Design review of the part built by this model. Coordinates are the model's own, in mm. A direction names the side the tool comes from. Coordinates: 2 decimals unless noted, no trailing zeros. Write each loop counter-clockwise with the first axis right and the second up, starting at its lowest first coordinate (ties: lowest second). Pieces come first, ordered by that corner, then holes. Notation, with made-up numbers: (-20.75, 2) - (-0.75, 2) arc R12 ccw to (-0.75, 11) - close; hole circle Ø1 at (71, 45). An arc over 180 degrees is marked (long way). One line per item, written item: value.
from build123d import *

# Parameters (mm, degrees)
ESBO_O1_W                  = 27
ESBO_O1_H                  = 75
RESSALTO_EXTRUS_O1_DEPTH   = 2
ESBO_O2_W                  = 75
ESBO_O2_H                  = 104
RESSALTO_EXTRUS_O2_DEPTH   = 2
ESBO_O3_W                  = 29
ESBO_O3_H                  = 75
RESSALTO_EXTRUS_O3_DEPTH   = 2
ESBO_O4_R                  = 5
CORTE_EXTRUS_O1_DEPTH      = 2
ESBO_O5_R                  = 2.5
CORTE_EXTRUS_O2_DEPTH      = 1
CORTE_EXTRUS_O2_DEPTH_BACK = 107
ESBO_O7_R                  = 3.5
CORTE_EXTRUS_O3_DEPTH      = 10


with BuildPart() as part:
    # Esboço1 → Ressalto-extrusão1 (new body)
    with BuildSketch(Plane(origin=(0, 0, 0), x_dir=(1, 0, 0), z_dir=(0, 1, 0))):
        Rectangle(ESBO_O1_W, ESBO_O1_H)
    extrude(amount=RESSALTO_EXTRUS_O1_DEPTH)

    # Esboço2 → Ressalto-extrusão2 (add)
    with BuildSketch(Plane.ZY.offset(13.5)):
        with Locations((0, 52)):
            Rectangle(ESBO_O2_W, ESBO_O2_H)
    extrude(amount=RESSALTO_EXTRUS_O2_DEPTH)

    # Esboço3 → Ressalto-extrusão3 (add)
    with BuildSketch(Plane(origin=(0, 104, 0), x_dir=(1, 0, 0), z_dir=(0, 1, 0))):
        with Locations((-1, 0)):
            Rectangle(ESBO_O3_W, ESBO_O3_H)
    extrude(amount=RESSALTO_EXTRUS_O3_DEPTH)

    # Esboço4 → Corte-extrusão1 (cut)
    with BuildSketch(Plane.ZY.offset(15.5)):
        with Locations((5.625, 53)):
            Circle(ESBO_O4_R)
    extrude(amount=-CORTE_EXTRUS_O1_DEPTH, mode=Mode.SUBTRACT)

    # Esboço5 → Corte-extrusão2 (cut, two sides)
    with BuildSketch(Plane(origin=(0, 106, 0), x_dir=(1, 0, 0), z_dir=(0, 1, 0))) as corte_extrus_o2_sk:
        with Locations((0, 27.5)):
            Circle(ESBO_O5_R)
        with Locations((0, -12.5)):
            Circle(ESBO_O5_R)
    extrude(amount=CORTE_EXTRUS_O2_DEPTH, mode=Mode.SUBTRACT)
    extrude(corte_extrus_o2_sk.sketch, amount=-CORTE_EXTRUS_O2_DEPTH_BACK, mode=Mode.SUBTRACT)

    # Esboço7 → Corte-extrusão3 (cut)
    with BuildSketch(Plane.ZY.offset(15.5)):
        with Locations((5.625, 75.5)):
            Circle(ESBO_O7_R)
        with Locations((5.625, 30.5)):
            Circle(ESBO_O7_R)
    extrude(amount=-CORTE_EXTRUS_O3_DEPTH, mode=Mode.SUBTRACT)


solid = part.part
1. Mouldability with a two-part tool opening along X and no side actions: class faces 3 (the face through (-0.54, 1.01, 14.94)), 4 (the face through (-1, 106, -1)), 5 (the face through (-15.5, 52.3, 0.5)) as released by +X, released by -X, zero draft, split by the parting line, or undercut.
Answer block:
face 3: undercut
face 4: zero draft
face 5: released by -X
2. Consider section A-A, the plane z = -27.5. Write out the cut boundary in (x, y), then the cut area to 3 significant figures.
Answer block:
outline: (-15.5, 0) - (-2.5, 0) - (-2.5, 2) - (-13.5, 2) - (-13.5, 104) - (-2.5, 104) - (-2.5, 106) - (-15.5, 106) - close; (2.5, 0) - (13.5, 0) - (13.5, 2) - (2.5, 2) - close; (2.5, 104) - (13.5, 104) - (13.5, 106) - (2.5, 106) - close
area: 300 mm^2
3. Insertion check: pin 1 Ø1 at (y, z) = (25, 29) entering from +X. The pin has a flat end and moves straight along its axis. Give the tip position at first contact, or say it passes through.
Answer block:
pin 1: stops at x = -13.5
4. For faces 1 (the face through (-14, 37, 37.5)), 2 (the face through (-13.5, 54, -1)), list the 3-axis set-ups (+Z, -Z, +X, -X, +Y, -Y) from which the entire face can be reached by the end or side of a thin tool; tool diameter is ignored.
Answer block:
face 1: +Z, +X, -X, +Y, -Y
face 2: +Z, -Z, +X
5. Consider section C-C, the plane x = 0. Write out the cut boundary in (y, z), then the cut area to 3 significant figures.
Answer block:
outline: (0, -37.5) - (2, -37.5) - (2, -30) - (0, -30) - close; (0, -25) - (2, -25) - (2, 10) - (0, 10) - close; (0, 15) - (2, 15) - (2, 37.5) - (0, 37.5) - close; (104, -37.5) - (106, -37.5) - (106, -30) - (104, -30) - close; (104, -25) - (106, -25) - (106, 10) - (104, 10) - close; (104, 15) - (106, 15) - (106, 37.5) - (104, 37.5) - close
area: 260 mm^2
6. Consider section B-B, the plane y = 30.5. Write out the cut boundary in (x, z) (3 decimals).
Answer block:
outline: (-15.5, -37.5) - (-13.5, -37.5) - (-13.5, 2.125) - (-15.5, 2.125) - close; (-15.5, 9.125) - (-13.5, 9.125) - (-13.5, 37.5) - (-15.5, 37.5) - close
7. Wall thickness on line 1 along Y through (x, z) = (-2.25, 27); line 2 along X through (y, z) = (1.2, -27.5); line 3 along X through (y, z) = (70.5, -17): over which ranges is each line inside the solid? List them lowest first.
Answer block:
line 1: y = 0 to 2, 104 to 106
line 2: x = -15.5 to -2.5, 2.5 to 13.5
line 3: x = -15.5 to -13.5
8. Consider section D-D, the plane x = -10. Write out the cut boundary in (y, z).
Answer block:
outline: (0, -37.5) - (2, -37.5) - (2, 37.5) - (0, 37.5) - close; (104, -37.5) - (106, -37.5) - (106, 37.5) - (104, 37.5) - close
